```python
from build123d import *

# Parameters (mm, degrees)
F0_R     = 25.4
F1_DEPTH = 25.4
F2_R     = 12.495543
F3_DEPTH = 43.18
F4_T     = -2.54


with BuildPart() as f1:
    # F0 (on Top) → F1 (new body, symmetric)
    with BuildSketch(Plane.XY):
        Circle(F0_R)
    extrude(amount=F1_DEPTH, both=True)

    # F2 (on Right) → F3 (cut, symmetric)
    with BuildSketch(Plane.YZ):
        Circle(F2_R)
    extrude(amount=F3_DEPTH, both=True, mode=Mode.SUBTRACT)

    # F4
    f4_openings = [f1.faces().sort_by_distance(p)[0] for p in [
        (0, 0, 25.4),
        (0, 0, -25.4),
    ]]
    offset(amount=F4_T, openings=f4_openings)


solid = f1.part
```
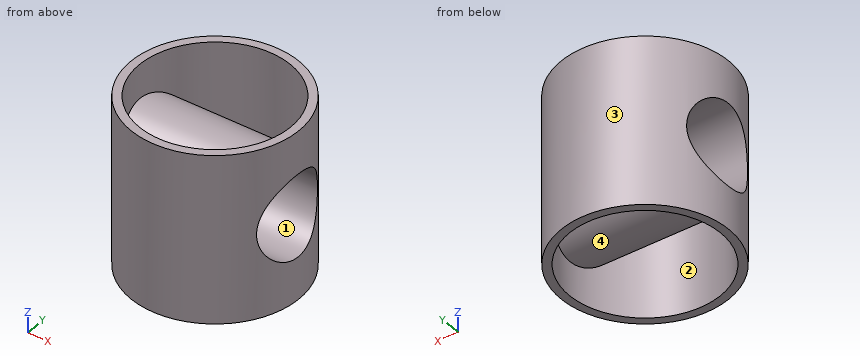
Design review of the part built by this model. Coordinates are the model's own, in mm. Face numbers are marked on the shaded views. A direction names the side the tool comes from. Give positions to 0.01 mm unless a question says otherwise; leave off trailing zeros. Loops run counter-clockwise (first coordinate to the right, second up) from the corner with the lowest first, then second, coordinate; pieces in that order, holes last. Notation, with made-up numbers: (26.5, 54) -> (38.5, 54) arc R25 cw to (38.5, 82) -> close; hole circle Ø4 at (79, 72.5). An arc over 180 degrees is marked (long way). One line per item, written item: value.
Q1. For L1, parallel to Y at x = 0.5, z = 0; L2, parallel to Y at x = 0, z = 13; L3, parallel to Y at x = 8, z = 13, list the stretches that pass through material, from the lowest coordinate up.
Numbers:
L1: y = -25.4 to -22.85, -15.04 to -12.5, 12.5 to 15.04, 22.85 to 25.4
L2: y = -25.4 to -22.86, -7.55 to 7.55, 22.86 to 25.4
L3: y = -24.11 to -21.41, -7.55 to 7.55, 21.41 to 24.11
Q2. We need section D-D on x = -20.5. Give the boundary of the cut face in (y, z), and give its area (3 significant figures).
Numbers:
outline: (-15, -25.4) -> (-10.12, -25.4) -> (-10.12, -11.12) arc R15.04 ccw to (10.12, -11.12) -> (10.12, -25.4) -> (15, -25.4) -> (15, 25.4) -> (10.12, 25.4) -> (10.12, 11.12) arc R15.04 ccw to (-10.12, 11.12) -> (-10.12, 25.4) -> (-15, 25.4) -> close; hole circle Ø24.99 at (0, 0)
area: 564 mm^2
Q3. Machinability: for the marked faces 1 and 2, which of the approach directions +Z, -Z, +X, -X, +Y, -Y give a long, thin tool a straight path to every point of the face, cutting with its end or side? Answer none if there is none.
Numbers:
face 1: +X, -X
face 2: none
Q4. For pin 1 Ø15 at (y, z) = (0, 0) entering from +X; pin 2 Ø1 at (x, y) = (-10, -1) entering from -Z; pin 3 Ø12 at (x, y) = (4.5, 16) entering from -Z; pin 4 Ø4 at (x, y) = (13.5, -12.5) entering from +Z, all flat-tipped, find the tip position at first contact; note any pin that passes through.
Numbers:
pin 1: passes through
pin 2: stops at z = -15.03
pin 3: stops at z = -11.23
pin 4: stops at z = 10.76
Q5. We need section C-C on x = -13. Give the boundary of the cut face in (y, z), and give its area (3 significant figures).
Numbers:
outline: (-21.82, -25.4) -> (-18.8, -25.4) -> (-18.8, 25.4) -> (-21.82, 25.4) -> close; circle Ø30.07 at (0, 0); (18.8, -25.4) -> (21.82, -25.4) -> (21.82, 25.4) -> (18.8, 25.4) -> close; hole circle Ø24.99 at (0, 0)
area: 526 mm^2
Q6. We need section B-B on z = 3. Give the boundary of the cut face in (x, y), and give its area (3 significant figures).
Numbers:
outline: (-22.32, -12.13) arc R25.4 ccw to (22.32, -12.13) -> close; (-22.32, 12.13) -> (22.32, 12.13) arc R25.4 ccw to start; hole (-17.48, -14.73) arc R22.86 ccw to (17.48, -14.73) -> close; hole (-17.48, 14.73) -> (17.48, 14.73) arc R22.86 ccw to start
area: 448 mm^2
Q7. We need section A-A on y = 0. Give the boundary of the cut face in (x, z).
Numbers:
outline: (-25.4, -25.4) -> (-22.86, -25.4) -> (-22.86, -15.04) -> (22.86, -15.04) -> (22.86, -25.4) -> (25.4, -25.4) -> (25.4, -12.5) -> (-25.4, -12.5) -> close; (-25.4, 12.5) -> (25.4, 12.5) -> (25.4, 25.4) -> (22.86, 25.4) -> (22.86, 15.04) -> (-22.86, 15.04) -> (-22.86, 25.4) -> (-25.4, 25.4) -> close
Q8. Draft analysis for pull direction Y (two halves, no side actions). For the marked faces 3 and 4, state which applies: pulls with the +Y half, pulls with the -Y half, needs draft (parallel to the pull), parting line crosses it, or undercut.
Numbers:
face 3: parting line crosses it
face 4: undercut
